Autodesk Inventor part; units mm, degrees
ref_plane "YZ Plane" through (0, 0, 0) normal (1, 0, 0) x (0, 1, 0)
ref_plane "XZ Plane" through (0, 0, 0) normal (0, 1, 0) x (-1, 0, 0)
ref_plane "XY Plane" through (0, 0, 0) normal (0, 0, 1) x (1, 0, 0)
sketch "Sketch1" plane through (0, 0, 0) normal (0, 0, 1) x (1, 0, 0)
  line L0 (-12.7, -25.4) -> (12.7, -25.4)
  line L1 (12.7, -25.4) -> (12.7, 25.4)
  line L2 (12.7, 25.4) -> (-12.7, 25.4)
  line L3 (-12.7, 25.4) -> (-12.7, -25.4)
  line L4 (-12.7, -25.4) -> (12.7, 25.4) construction
  line L5 (12.7, -25.4) -> (-12.7, 25.4) construction
  line L6 (-11.1125, 23.8125) -> (11.1125, 23.8125)
  line L7 (11.1125, 23.8125) -> (11.1125, -23.8125)
  line L8 (11.1125, -23.8125) -> (-11.1125, -23.8125)
  line L9 (-11.1125, -23.8125) -> (-11.1125, 23.8125)
  point P0 (0, 0)
  dimension "width" = 25.4
  dimension "height" = 50.8
  dimension "thickness" = 1.5875
extrude "Extrusion1" add sketch "Sketch1" along normal mid plane 152.4
sketch "Sketch2" plane through (-12.7, 25.4, 76.2) normal (0, 1, 0) x (1, 0, 0)
  line L0 (25.4, 0) -> (0, 0) construction
  line L1 (0, 152.4) -> (0, 0) construction
  line L2 (25.4, 0) -> (0, 0) construction
  line L3 (25.4, 152.4) -> (25.4, 0) construction
  line L4 (0, 152.4) -> (25.4, 152.4) construction
  point P0 (12.7, 76.2)
  point P1 (12.7, 12.7)
  point P2 (12.7, 25.4)
  point P3 (12.7, 38.1)
  point P4 (12.7, 50.8)
  point P5 (12.7, 63.5)
  point P6 (12.7, 76.2)
  point P7 (12.7, 88.9)
  point P8 (12.7, 101.6)
  point P9 (12.7, 114.3)
  point P10 (12.7, 127)
  point P11 (12.7, 139.7)
  dimension "d5" = 12.7
  dimension "d8" = 12.7
hole "Hole1" at (0, 25.4, 63.5) at (0, 25.4, 50.8) at (0, 25.4, 38.1) at (0, 25.4, 25.4) at (0, 25.4, 12.7) at (0, 25.4, 0) at (0, 25.4, -12.7) at (0, 25.4, -25.4) at (0, 25.4, -38.1) at (0, 25.4, -50.8) at (0, 25.4, -63.5) direction (0, -1, 0) diameter 5.1054 end through all
sketch "Sketch3" plane through (12.7, -25.4, 76.2) normal (1, 0, 0) x (0, 0, -1)
  line L0 (6.35, 38.1) -> (6.35, 12.7) construction
  line L1 (0, 0) -> (0, 50.8) construction
  line L2 (152.4, 50.8) -> (0, 50.8) construction
  line L3 (0, 0) -> (0, 50.8) construction
  line L4 (152.4, 0) -> (0, 0) construction
  line L5 (152.4, 50.8) -> (152.4, 0) construction
  point P0 (76.2, 25.4)
  point P1 (6.35, 25.4)
  point P2 (19.05, 38.1)
  point P3 (19.05, 12.7)
  point P4 (31.75, 38.1)
  point P5 (31.75, 12.7)
  point P6 (44.45, 38.1)
  point P7 (44.45, 12.7)
  point P8 (57.15, 38.1)
  point P9 (57.15, 12.7)
  point P10 (69.85, 38.1)
  point P11 (69.85, 12.7)
  point P12 (82.55, 38.1)
  point P13 (82.55, 12.7)
  point P14 (95.25, 38.1)
  point P15 (95.25, 12.7)
  point P16 (107.95, 38.1)
  point P17 (107.95, 12.7)
  point P18 (120.65, 38.1)
  point P19 (120.65, 12.7)
  point P20 (133.35, 38.1)
  point P21 (133.35, 12.7)
  point P22 (146.05, 38.1)
  point P23 (146.05, 12.7)
  dimension "d20" = 25.4
  dimension "d21" = 6.35
  dimension "d24" = 12.7
hole "Hole2" at (12.7, 12.7, 69.85) at (12.7, -12.7, 69.85) at (12.7, 12.7, 57.15) at (12.7, -12.7, 57.15) at (12.7, 12.7, 44.45) at (12.7, -12.7, 44.45) at (12.7, 12.7, 31.75) at (12.7, -12.7, 31.75) at (12.7, 12.7, 19.05) at (12.7, -12.7, 19.05) at (12.7, 12.7, 6.35) at (12.7, -12.7, 6.35) at (12.7, 12.7, -6.35) at (12.7, -12.7, -6.35) at (12.7, 12.7, -19.05) at (12.7, -12.7, -19.05) at (12.7, 12.7, -31.75) at (12.7, -12.7, -31.75) at (12.7, 12.7, -44.45) at (12.7, -12.7, -44.45) at (12.7, 12.7, -57.15) at (12.7, -12.7, -57.15) at (12.7, 12.7, -69.85) at (12.7, -12.7, -69.85) direction (-1, 0, 0) diameter 5.1054 end through all
properties part number "CL7-006" material "Aluminum 6061"
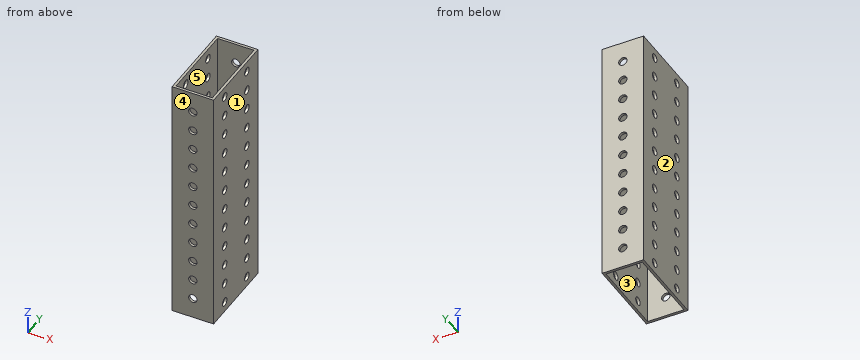
The listing builds one solid part. Answer for the finished solid, in the listing's coordinates (mm). Face numbers are marked on the shaded views. A direction names the side the tool comes from. Round coordinates to 2 decimals unless told otherwise and drop trailing zeros. Loops run counter-clockwise (first coordinate to the right, second up) from the corner with the lowest first, then second, coordinate; pieces in that order, holes last. Notation, with made-up numbers: (19, 78.25) - (24, 78.25) arc R32 cw to (24, 106.25) - close; hole circle Ø4 at (-10, -24.75). An arc over 180 degrees is marked (long way). Return JSON: item names as keys, results as strings. Group by question number.
1. The part is cut by section C-C on y = -4. Determine the outline of the cut face in (x, z), then the cut area to 3 significant figures.
2. The part is cut by section A-A on z = 38.1. Determine the outline of the cut face in (x, y), then the cut area to 3 significant figures.
3. Which of the six approach directions +Z, -Z, +X, -X, +Y, -Y give full straight-line access (tool end or side, diameter ignored) to the marked faces 4 and 5?
4. The part is cut by section D-D on z = 69.85. Determine the outline of the cut face in (x, y).
5. This flat-tipped pin is pushed along its axis until it touches: P1, Ø4.5, axis at x = 0, z = 12.7, coming from the -Y side. Where does it stop, or does it pass through?
6. The mould has two halves that part along X. Classify the marked faces 1, 2 and 3: pulls with the +X half, pulls with the -X half, needs draft (parallel to the pull), parting line crosses it, or undercut.
7. Consider probe 1 along Y at (x, z) = (11.65, 6.35); probe 2 along X at (y, z) = (-9.5, -33); probe 3 along Y at (x, z) = (-8, 17). Determine where each line is inside the solid, lowest interval first.
8. The part is cut by section B-B on x = -5.75. Determine the outline of the cut face in (y, z).
Resolved:
{
 "1": {"outline": "(-12.7, -76.2) - (-11.11, -76.2) - (-11.11, 76.2) - (-12.7, 76.2) - close; (11.11, -76.2) - (12.7, -76.2) - (12.7, 76.2) - (11.11, 76.2) - close", "area": "484 mm²"},
 "2": {"outline": "(-12.7, -25.4) - (-2.55, -25.4) - (-2.55, -23.81) - (-11.11, -23.81) - (-11.11, 23.81) - (-2.55, 23.81) - (-2.55, 25.4) - (-12.7, 25.4) - close; (2.55, -25.4) - (12.7, -25.4) - (12.7, 25.4) - (2.55, 25.4) - (2.55, 23.81) - (11.11, 23.81) - (11.11, -23.81) - (2.55, -23.81) - close", "area": "216 mm²"},
 "3": {"face 4": "+Z, -Z, +X, -X, -Y", "face 5": "+Z, -Z"},
 "4": {"outline": "(-12.7, -25.4) - (12.7, -25.4) - (12.7, -15.25) - (11.11, -15.25) - (11.11, -23.81) - (-11.11, -23.81) - (-11.11, -15.25) - (-12.7, -15.25) - close; (-12.7, -10.15) - (-11.11, -10.15) - (-11.11, 10.15) - (-12.7, 10.15) - close; (-12.7, 15.25) - (-11.11, 15.25) - (-11.11, 23.81) - (11.11, 23.81) - (11.11, 15.25) - (12.7, 15.25) - (12.7, 25.4) - (-12.7, 25.4) - close; (11.11, -10.15) - (12.7, -10.15) - (12.7, 10.15) - (11.11, 10.15) - close"},
 "5": {"P1": "passes through"},
 "6": {"face 1": "pulls with the +X half", "face 2": "pulls with the -X half", "face 3": "undercut"},
 "7": {"probe 1": "y = -25.4 to -15.25, -10.15 to 10.15, 15.25 to 25.4", "probe 2": "x = -12.7 to -11.11, 11.11 to 12.7", "probe 3": "y = -25.4 to -23.81, 23.81 to 25.4"},
 "8": {"outline": "(-25.4, -76.2) - (-23.81, -76.2) - (-23.81, 76.2) - (-25.4, 76.2) - close; (23.81, -76.2) - (25.4, -76.2) - (25.4, 76.2) - (23.81, 76.2) - close"}
}
